Answer from the drawing. Dimensions are ordinates in mm from the lowest x, y and z of the part. A direction names the side the tool comes from. Give positions to 0.01 mm unless a question says otherwise; leave off trailing zeros. Answer as a JSON object with one key per item and string values.
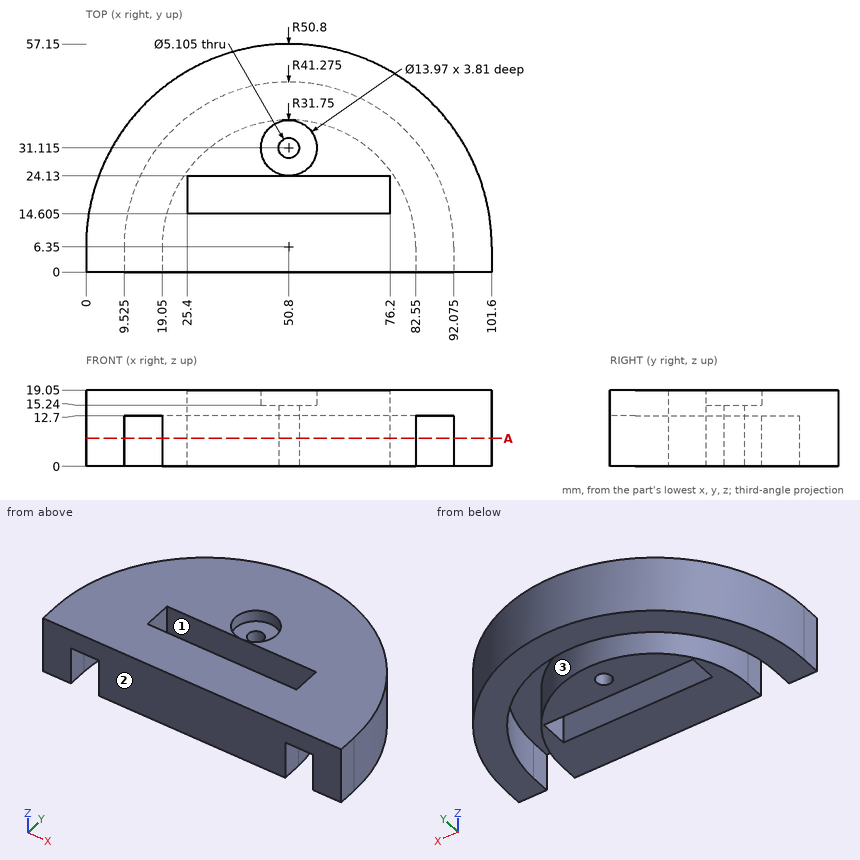
1. A cutting plane is placed at A-A, the plane z = 7. Count the separate pieces of the cut face and the enclosed holes in it, plus the area to 3 significant figures.
Verdict:
{"separate pieces": "2", "enclosed holes": "2", "area": "2,980 mm2"}
2. Consider line 1 along X through (y, z) = (11.5, 10.5); line 2 along Y through (x, z) = (30, 1.75) (1 decimal); line 3 along Y through (x, z) = (28, 11) (1 decimal). Determine where each line is inside the solid, lowest interval first.
Verdict:
{"line 1": "x = 0.26 to 9.85, 19.47 to 82.13, 91.75 to 101.34", "line 2": "y = 0 to 14.6, 24.1 to 30.3, 42 to 52.7", "line 3": "y = 0 to 14.6, 24.1 to 28.4, 40.8 to 51.7"}
3. For the marked faces 1, 2 and 3, determine the directions among +Z, -Z, +X, -X, +Y, -Y from which every point of the face is accessible in a straight line to the end or side of a thin tool.
Verdict:
{"face 1": "+Z, -Z", "face 2": "+Z, -Z, +X, -X, -Y", "face 3": "-Z"}
4. Flat-ended cylindrical pins translate along their axes: pin 1 (9.5 mm diameter, centred on x = 62, z = 11, fed in from +Y); pin 2 (3 mm diameter, centred on x = 38, z = 5.5, fed in from +Y); pin 3 (3 mm diameter, centred on y = 19, z = 8, fed in from -X). Find the tip coordinate at first contact, or state that the pin passes through.
Verdict:
{"pin 1": "stops at y = 56.74", "pin 2": "stops at y = 55.88", "pin 3": "stops at x = 1.24"}
